Source: CAD feature listing. Evaluate the final solid. Frame: model axes, mm. Face numbers are marked on the shaded views. A direction names the side the tool comes from. Coordinates: 2 decimals unless noted, no trailing zeros. Write each loop counter-clockwise with the first axis right and the second up, starting at its lowest first coordinate (ties: lowest second). Pieces come first, ordered by that corner, then holes. Notation, with made-up numbers: M -16,79.5 L 9,79.5 A23 cw 9,90.5 Z; hole C -0.75,-16.5 d8. An arc over 180 degrees is marked long. Write item = value, one per line. Start each with the question number.
1. Section query A-A (z = 5). Output: boundary loops of the cut face in (x, y), then the cut area to 3 significant figures.
2. Access query for the marked faces 1, 2 and 3. Directions: +Z, -Z, +X, -X, +Y, -Y. A direction counts if a zero-diameter tool reaches every point of the face in a straight line with its end or side. Return the directions, or none.
3. Section query B-B (x = 10.5). Give the number of separate pieces and of enclosed holes in the cut face, then the cut area to 3 significant figures.
4. Line query: line 1 along Z through (x, y) = (25.8, 5.5); line 2 along Z through (x, y) = (17.83, 18.45); line 3 along Z through (x, y) = (24, 11). Output: solid intervals per line, ascending.
5. Pin query (flat end, axial travel): pin 1 Ø8.5 at (x, z) = (17.83, 31.04) entering from -Y; pin 2 Ø1.2 at (y, z) = (0.5, 12.5) entering from -X. Return the tip coordinate at first contact, or that it passes through.
6. Pull-direction query (Z, two-part tool) for the marked faces 4, 5 and 6; classes: pulls with the +Z half, pulls with the -Z half, needs draft (parallel to the pull), parting line crosses it, or undercut.
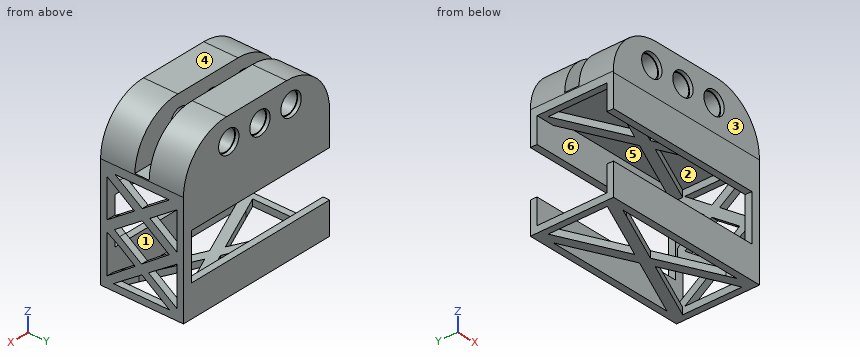
```python
from build123d import *

# Parameters (mm, degrees)
SKETCH1_W            = 37.4
SKETCH1_H            = 18.8
BOSS_EXTRUDE1_DEPTH  = 2
SKETCH2_W            = 33.4
SKETCH2_H            = 15.8
BOSS_EXTRUDE2_DEPTH  = 23
SKETCH4_W            = 22
SKETCH4_H            = 15.8
CUT_EXTRUDE3_DEPTH   = 5550
SKETCH6_W            = 34.4
SKETCH6_H            = 15.8
CUT_EXTRUDE4_DEPTH   = 5550
CUT_EXTRUDE5_DEPTH   = 5550
BOSS_EXTRUDE3_DEPTH  = 1.5
BOSS_EXTRUDE4_DEPTH  = 1.5
BOSS_EXTRUDE5_DEPTH  = 1.5
SKETCH11_W           = 35.4
SKETCH11_H           = 5.25
BOSS_EXTRUDE6_DEPTH  = 1.5
SKETCH12_W           = 35.4
SKETCH12_H           = 7.25
BOSS_EXTRUDE7_DEPTH  = 1.5
SKETCH13_W           = 35.4
SKETCH13_H           = 5.25
BOSS_EXTRUDE8_DEPTH  = 1.5
SKETCH14_W           = 35.4
SKETCH14_H           = 5.25
BOSS_EXTRUDE9_DEPTH  = 1.5
SKETCH15_W           = 37.4
SKETCH15_H           = 2.35
BOSS_EXTRUDE10_DEPTH = 1.5
SKETCH16_W           = 37.4
SKETCH16_H           = 2.35
CUT_EXTRUDE6_DEPTH   = 10
SKETCH17_W           = 37.4
SKETCH17_H           = 11.3
SKETCH17_R           = 2.4
BOSS_EXTRUDE11_DEPTH = 18.76
FILLET2_R            = 11
FILLET3_R            = 11
SKETCH21_W           = 41.68561835
SKETCH21_H           = 3.24
CUT_EXTRUDE7_DEPTH   = 10.76
SKETCH22_R           = 2.6
CUT_EXTRUDE8_DEPTH   = 0.8
SKETCH23_R           = 2.6
CUT_EXTRUDE9_DEPTH   = 0.8


with BuildPart() as part:
    # Sketch1 → Boss-Extrude1 (new body)
    with BuildSketch(Plane.XY):
        with Locations((18.7, 9.4)):
            Rectangle(SKETCH1_W, SKETCH1_H)
    extrude(amount=BOSS_EXTRUDE1_DEPTH)

    # Sketch2 → Boss-Extrude2 (add)
    with BuildSketch(Plane.XY.offset(2)):
        Polygon((0, 18.8), (37.4, 18.8), (37.4, 17.3), (37.4, 0), (0, 0), (0, 16.8), align=None)
        with Locations((18.7, 9.4)):
            Rectangle(SKETCH2_W, SKETCH2_H, mode=Mode.SUBTRACT)
    extrude(amount=BOSS_EXTRUDE2_DEPTH)

    # Sketch4 → Cut-Extrude3 (cut)
    with BuildSketch(Plane.ZY):
        with Locations((12.5, 9.4)):
            Rectangle(SKETCH4_W, SKETCH4_H)
    extrude(amount=-CUT_EXTRUDE3_DEPTH, mode=Mode.SUBTRACT)

    # Sketch6 → Cut-Extrude4 (cut)
    with BuildSketch(Plane(origin=(0, 0, 0), x_dir=(-1, 0, 0), z_dir=(0, 0, -1))):
        with Locations((-18.7, 9.4)):
            Rectangle(SKETCH6_W, SKETCH6_H)
    extrude(amount=-CUT_EXTRUDE4_DEPTH, mode=Mode.SUBTRACT)

    # Sketch7 → Cut-Extrude5 (cut)
    with BuildSketch(Plane(origin=(0, 18.8, 0), x_dir=(1, 0, 0), z_dir=(0, 1, 0))):
        Polygon((1.635040334, -2), (35.4, -2), (35.4, -23), (1.635040334, -23), (0, -23), (0, -2), align=None)
    extrude(amount=-CUT_EXTRUDE5_DEPTH, mode=Mode.SUBTRACT)

    # Sketch8 → Boss-Extrude3 (add)
    with BuildSketch(Plane(origin=(0, 0, 0), x_dir=(-1, 0, 0), z_dir=(0, 0, -1))):
        Polygon((-35.9, 16.089041374), (-35.9, 17.3), (-33.263482485, 17.3), (-18.638089895, 10.582523171), (-4.136517515, 17.3), (-1.5, 17.3), (-1.5, 16.089041374), (-16.074159281, 9.404903878), (-5.039195107, 4.33651917), (-1.5, 2.710958626), (-1.5, 1.5), (-4.136517515, 1.5), (-5.957799758, 2.33651917), (-18.712609683, 8.194833031), (-31.486134971, 2.33651917), (-33.263482485, 1.5), (-35.9, 1.5), (-35.9, 2.710958626), (-32.318884833, 4.245250178), (-21.26339944, 9.366416698), align=None)
    extrude(amount=-BOSS_EXTRUDE3_DEPTH)

    # Sketch9 → Boss-Extrude4 (add)
    with BuildSketch(Plane.XY.offset(25)):
        Polygon((21.336517515, 9.4), (35.9, 16.089041374), (35.9, 17.3), (33.263482485, 17.3), (18.7, 10.610958626), (4.136517515, 17.3), (1.5, 17.3), (1.5, 16.089041374), (16.063482485, 9.4), (1.5, 2.710958626), (1.5, 1.5), (4.136517515, 1.5), (18.7, 8.189041374), (33.263482485, 1.5), (35.9, 1.5), (35.9, 2.710958626), align=None)
    extrude(amount=-BOSS_EXTRUDE4_DEPTH)

    # Sketch10 → Boss-Extrude5 (add)
    with BuildSketch(Plane(origin=(37.4, 0, 0), x_dir=(0, 0, -1), z_dir=(1, 0, 0))):
        Polygon((-23.5, 17.3), (-23.5, 15.627431355), (-19.218481828, 9.477614344), (-22.771372102, 4.374371951), (-23.5, 3.327797334), (-23.5, 1.5), (-22.335553475, 1.5), (-21.129985293, 3.231634299), (-18, 7.727431355), (-14.870014707, 3.231634299), (-13.664446525, 1.5), (-12.445964697, 1.5), (-11.227482869, 1.5), (-9.490525788, 4.374371951), (-7.004939959, 7.874823075), (-4.491504582, 4.374371951), (-2.427613988, 1.5), (-1.5, 1.5), (-1.5, 2.993507593), (-2.491504582, 4.374371951), (-5.926135142, 9.394104162), (-1.5, 15.627431355), (-1.5, 17.3), (-2.491504582, 17.3), (-6.951935611, 10.893317416), (-11.335553475, 17.3), (-13.772517131, 17.3), (-18, 11.227797334), (-22.227482869, 17.3), align=None)
        Polygon((-11.490525788, 4.374371951), (-12.395540567, 3.177755602), (-13.228627898, 4.374371951), (-16.781518172, 9.477614344), (-12.535227515, 15.576831834), (-8.044999313, 9.323309465), align=None, mode=Mode.SUBTRACT)
    extrude(amount=-BOSS_EXTRUDE5_DEPTH)

    # Sketch11 → Boss-Extrude6 (add)
    with BuildSketch(Plane(origin=(0, 18.8, 0), x_dir=(1, 0, 0), z_dir=(0, 1, 0))):
        with Locations((17.7, -4.625)):
            Rectangle(SKETCH11_W, SKETCH11_H)
    extrude(amount=-BOSS_EXTRUDE6_DEPTH)

    # Sketch12 → Boss-Extrude7 (add)
    with BuildSketch(Plane(origin=(0, 18.8, 0), x_dir=(1, 0, 0), z_dir=(0, 1, 0))):
        with Locations((17.7, -21.375)):
            Rectangle(SKETCH12_W, SKETCH12_H)
    extrude(amount=-BOSS_EXTRUDE7_DEPTH)

    # Sketch13 → Boss-Extrude8 (add)
    with BuildSketch(Plane.XZ):
        with Locations((17.7, 20.375)):
            Rectangle(SKETCH13_W, SKETCH13_H)
    extrude(amount=-BOSS_EXTRUDE8_DEPTH)

    # Sketch14 → Boss-Extrude9 (add)
    with BuildSketch(Plane.XZ):
        with Locations((17.7, 4.625)):
            Rectangle(SKETCH14_W, SKETCH14_H)
    extrude(amount=-BOSS_EXTRUDE9_DEPTH)

    # Sketch15 → Boss-Extrude10 (add)
    with BuildSketch(Plane(origin=(0, 18.8, 0), x_dir=(1, 0, 0), z_dir=(0, 1, 0))):
        with Locations((18.7, 1.175)):
            Rectangle(SKETCH15_W, SKETCH15_H)
    extrude(amount=-BOSS_EXTRUDE10_DEPTH)

    # Sketch16 → Cut-Extrude6 (cut)
    with BuildSketch(Plane(origin=(0, 18.8, 0), x_dir=(1, 0, 0), z_dir=(0, 1, 0))):
        with Locations((18.7, 1.175)):
            Rectangle(SKETCH16_W, SKETCH16_H)
    extrude(amount=-CUT_EXTRUDE6_DEPTH, mode=Mode.SUBTRACT)

    # Sketch17 → Boss-Extrude11 (add)
    with BuildSketch(Plane(origin=(0, 18.8, 0), x_dir=(1, 0, 0), z_dir=(0, 1, 0))):
        with Locations((18.7, -30.65)):
            Rectangle(SKETCH17_W, SKETCH17_H)
        with Locations((25.8, -31.04)):
            Circle(SKETCH17_R, mode=Mode.SUBTRACT)
        with Locations((17.83, -31.04)):
            Circle(SKETCH17_R, mode=Mode.SUBTRACT)
        with Locations((9.86, -31.04)):
            Circle(SKETCH17_R, mode=Mode.SUBTRACT)
    extrude(amount=-BOSS_EXTRUDE11_DEPTH)

    # Fillet2
    fillet2_edges = [part.edges().sort_by_distance(p)[0] for p in [
        (0, 9.42, 36.3),
    ]]
    fillet(fillet2_edges, radius=FILLET2_R)

    # Fillet3
    fillet3_edges = [part.edges().sort_by_distance(p)[0] for p in [
        (37.4, 9.42, 36.3),
    ]]
    fillet(fillet3_edges, radius=FILLET3_R)

    # Sketch21 → Cut-Extrude7 (cut)
    with BuildSketch(Plane.XY.offset(36.3)):
        with Locations((18.29957708, 9.42)):
            Rectangle(SKETCH21_W, SKETCH21_H)
    extrude(amount=-CUT_EXTRUDE7_DEPTH, mode=Mode.SUBTRACT)

    # Sketch22 → Cut-Extrude8 (cut)
    with BuildSketch(Plane.XZ.offset(-0.04)):
        with Locations((9.86, 31.04)):
            Circle(SKETCH22_R)
        with Locations((17.83, 31.04)):
            Circle(SKETCH22_R)
        with Locations((25.8, 31.04)):
            Circle(SKETCH22_R)
    extrude(amount=-CUT_EXTRUDE8_DEPTH, mode=Mode.SUBTRACT)

    # Sketch23 → Cut-Extrude9 (cut)
    with BuildSketch(Plane(origin=(0, 18.8, 0), x_dir=(1, 0, 0), z_dir=(0, 1, 0))):
        with Locations((9.86, -31.04)):
            Circle(SKETCH23_R)
        with Locations((17.83, -31.04)):
            Circle(SKETCH23_R)
        with Locations((25.8, -31.04)):
            Circle(SKETCH23_R)
    extrude(amount=-CUT_EXTRUDE9_DEPTH, mode=Mode.SUBTRACT)


solid = part.part
```
Results are:
q1.outline = M 0,0 L 37.4,0 L 37.4,1.5 L 0,1.5 Z; M 0,17.3 L 37.4,17.3 L 37.4,18.8 L 0,18.8 Z; M 35.9,5.08 L 37.4,5.08 L 37.4,8.04 L 35.9,8.04 Z; M 35.9,10.7 L 37.4,10.7 L 37.4,13.7 L 35.9,13.7 Z
q1.area = 121 mm^2
q2.face_1 = none
q2.face_2 = -Z
q2.face_3 = +Z, +X, -X, -Y
q3.separate_pieces = 7
q3.enclosed_holes = 0
q3.area = 162 mm^2
q4.line_1 = 0 to 1.5, 23.5 to 28.64, 33.44 to 36.3
q4.line_2 = 0 to 7.25, 17.75 to 28.44, 33.64 to 36.3
q4.line_3 = 0 to 1.5, 23.5 to 25.54
q5.pin_1 = 0.04
q5.pin_2 = 35.4
q6.face_4 = pulls with the +Z half
q6.face_5 = pulls with the -Z half
q6.face_6 = undercut
